Solid Edge part; units mm, degrees
sketch "Sketch1" plane through (0, 0, 0) normal (0, -1, 0) x (1, 0, 0)
  line L0 (0, 0) -> (0, 12.5)
  line L1 (0, 12.5) -> (10, 12.5)
  line L2 (10, 12.5) -> (10, 7.5)
  line L3 (10, 7.5) -> (14, 7.5)
  line L4 (14, 7.5) -> (14, 0)
revolve "RevolvedProtrusion1" add sketch "Sketch1" angle 360 about axis through (13.3633, 0, 0) along (-1, 0, 0)
sketch "Sketch2" plane through (0, 0, 0) normal (1, 0, 0) x (0, 1, 0)
  line L0 (12.5, 85) -> (12.5, 45)
  line L1 (6.25, 0) -> (12.5, 45)
  line L2 (-6.25, 0) -> (6.25, 0)
  line L3 (-6.25, 0) -> (-12.5, 45)
  line L4 (-12.5, 45) -> (-12.5, 85)
  line L5 (-12.5, 85) -> (12.5, 85)
  dimension "D1" = 6.25
  dimension "D2" = 12.5
extrude "Protrusion1" add sketch "Sketch2" along normal blind 9
hole "Hole_1" at (0, 0, 0) direction (1, 0, 0) diameter 4 end up to next
chamfer "Chamfer_1" distance 0.5 angle 60 1 edges at (14, 0, -7.5) measured on face at (14, -4.85, -5.15)
sketch "Sketch3" plane through (0, 0, 36.25) normal (-1, 0, 0) x (0, 0, 1)
  line L0 (48.75, 12.5) -> (48.75, -12.5)
  line L1 (48.75, -12.5) -> (36.25, -12.5)
  line L2 (36.25, -12.5) -> (36.25, 12.5)
  line L3 (36.25, 12.5) -> (48.75, 12.5)
extrude "ExtrudedCutout_1" cut sketch "Sketch3" against normal blind 4
hole "Hole_2" at (4, 5, 78.75) direction (1, 0, 0) diameter 5 end up to next
hole "Hole1" at (4, -5, 78.75) direction (1, 0, 0) diameter 5 end up to next
chamfer "Chamfer_2" distance 0.5 angle 60 1 edges at (0, 0, -2) measured on face at (0, -8.0833, 59.1833)
hole "Hole_4" at (0, 0, 50) direction (1, 0, 0) diameter 10 end up to next counterbore diameter 16 counterbore depth 5
properties material "Polyethylene, low density"
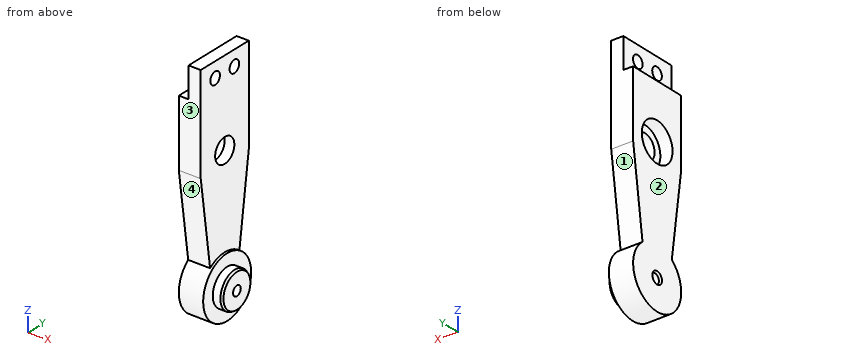
Build history of the part. All positions in model axes, mm. Face numbers are marked on the shaded views. A direction names the side the tool comes from. Give positions to 0.01 mm unless a question says otherwise; leave off trailing zeros. Loops run counter-clockwise (first coordinate to the right, second up) from the corner with the lowest first, then second, coordinate; pieces in that order, holes last. Notation, with made-up numbers: (-29.5, 21.5) -> (12.5, 21.5) arc R5 ccw to (12.5, 30.5) -> close; hole circle Ø3 at (71.5, -17.5). An arc over 180 degrees is marked (long way). One line per question, with ' | ' between items.
Q1. Drop flat-ended pins along their axis: pin 1 (11.5 mm diameter, centred on y = 0, z = 50, fed in from -X); pin 2 (7.5 mm diameter, centred on y = -5, z = 64.5, fed in from +X); pin 3 (3 mm diameter, centred on x = 6, y = 2, fed in from -Z). Give the stop position or say it passes through.
Filled sheet:
pin 1: stops at x = 5 | pin 2: stops at x = 9 | pin 3: stops at z = -12.49
Q2. Cut at A-A, the plane z = 78.75. Write the cut outline in (x, y), plus the area to 3 significant figures.
Filled sheet:
outline: (4, -12.5) -> (9, -12.5) -> (9, -7.5) -> (4, -7.5) -> close; (4, -2.5) -> (9, -2.5) -> (9, 2.5) -> (4, 2.5) -> close; (4, 7.5) -> (9, 7.5) -> (9, 12.5) -> (4, 12.5) -> close | area: 75.0 mm²
Q3. Cut at B-B, the plane x = 8. Write the cut outline in (y, z), plus the area to 3 significant figures.
Filled sheet:
outline: (-12.5, 45) -> (-7.63, 9.9) arc R12.5 ccw (long way) to (7.63, 9.9) -> (12.5, 45) -> (12.5, 85) -> (-12.5, 85) -> close; hole circle Ø5 at (-5, 78.75); hole circle Ø10 at (0, 50); hole circle Ø4 at (0, 0); hole circle Ø5 at (5, 78.75) | area: 2,040 mm²
Q4. Tool access for the marked faces 1 and 2: list every direction of +Z, -Z, +X, -X, +Y, -Y with a clear straight run to the whole face (end or side of a thin tool).
Filled sheet:
face 1: +X, -X, +Y | face 2: +Z, -Z, -X, +Y, -Y
Q5. Cut at C-C, the plane y = 0. Write the cut outline in (x, z), plus the area to 3 significant figures.
Filled sheet:
outline: (0, -12.5) -> (10, -12.5) -> (10, -7.5) -> (13.13, -7.5) -> (14, -7) -> (14, -2) -> (0.87, -2) -> (0, -2.5) -> close; (0, 2.5) -> (0.87, 2) -> (14, 2) -> (14, 7) -> (13.13, 7.5) -> (10, 7.5) -> (10, 12.5) -> (9, 12.5) -> (9, 45) -> (5, 45) -> (5, 42) -> (0, 42) -> close; (0, 58) -> (5, 58) -> (5, 55) -> (9, 55) -> (9, 85) -> (4, 85) -> (4, 72.5) -> (0, 72.5) -> close | area: 736 mm²
Q6. Cut at D-D, the plane z = 50. Write the cut outline in (x, y), plus the area to 3 significant figures.
Filled sheet:
outline: (0, -12.5) -> (9, -12.5) -> (9, -5) -> (5, -5) -> (5, -8) -> (0, -8) -> close; (0, 8) -> (5, 8) -> (5, 5) -> (9, 5) -> (9, 12.5) -> (0, 12.5) -> close | area: 105 mm²
Q7. Pull direction Z, two halves, no side cores. Call the marked faces 3 and 4: pulls with the +Z half, pulls with the -Z half, needs draft (parallel to the pull), parting line crosses it, or undercut.
Filled sheet:
face 3: needs draft | face 4: undercut
Q8. Drill centre lines: line 1 along Y through (x, z) = (5.65, 78.75); line 2 along Y through (x, z) = (3.05, 50); line 3 along Y through (x, z) = (5.25, 0). Where is each one in solid material? Low to high. Write a range as [from, to].
Filled sheet:
line 1: y = [-12.5, -7.5], [-2.5, 2.5], [7.5, 12.5] | line 2: y = [-12.5, -8], [8, 12.5] | line 3: y = [-12.5, -2], [2, 12.5]
